```python
from build123d import *

# Parameters (mm, degrees)
SKETCH_1_R           = 2
EXTRUDE_1_DEPTH      = 6
CHAMFER_3_SIZE       = 2
SKETCH_4_R           = 4.2
EXTRUDE_2_DEPTH      = 6
SKETCH_7_R           = 8
EXTRUDE_3_DEPTH      = 7
FILLET_1_R           = 2
EXTRUDE_4_DEPTH      = 3
EXTRUDE_4_DEPTH_BACK = 3
SKETCH_9_R           = 4.2
CUT_EXTRUDE_1_DEPTH  = 10


with BuildPart() as part:
    # Эскиз1 → Бобышка-Вытянуть1 (new body)
    with BuildSketch(Plane(origin=(0, 0, 0), x_dir=(1, 0, 0), z_dir=(0, 1, 0))):
        with BuildLine():
            Line((0, -20), (0, 20))
            Line((0, 20), (-10.861288353, 20))
            ThreePointArc((-10.861288353, 20), (-12.418498887, 19.751325642), (-13.820814088, 19.030038141))
            Line((-13.820814088, 19.030038141), (-34.246577377, 4.030038141))
            ThreePointArc((-34.246577377, 4.030038141), (-36.287051642, 0), (-34.246577377, -4.030038141))
            Line((-34.246577377, -4.030038141), (-13.820814088, -19.030038141))
            ThreePointArc((-13.820814088, -19.030038141), (-12.418498887, -19.751325642), (-10.861288353, -20))
            Line((-10.861288353, -20), (0, -20))
        make_face()
        with Locations((-31.287051642, 0)):
            Circle(SKETCH_1_R, mode=Mode.SUBTRACT)
        with Locations((-10.861288353, -15)):
            Circle(SKETCH_1_R, mode=Mode.SUBTRACT)
        with Locations((-10.861288353, 15)):
            Circle(SKETCH_1_R, mode=Mode.SUBTRACT)
    extrude(amount=EXTRUDE_1_DEPTH)

    # Фаска3
    chamfer_3_edges = [part.edges().sort_by_distance(p)[0] for p in [
        (-12.861288353, 6, -15),
        (-33.287051642, 6, 0),
        (-12.861288353, 6, 15),
    ]]
    chamfer(chamfer_3_edges, length=CHAMFER_3_SIZE)

    # Эскиз4 → Бобышка-Вытянуть2 (add)
    with BuildSketch(Plane(origin=(0, 0, 0), x_dir=(0, 0, -1), z_dir=(1, 0, 0))):
        with BuildLine():
            Line((-7.252328736, 33.376940613), (-20, 6))
            Line((-20, 6), (20, 6))
            Line((20, 6), (7.252328736, 33.376940613))
            ThreePointArc((7.252328736, 33.376940613), (0, 38), (-7.252328736, 33.376940613))
        make_face()
        with Locations((0, 30)):
            Circle(SKETCH_4_R, mode=Mode.SUBTRACT)
    extrude(amount=-EXTRUDE_2_DEPTH)

    # Эскиз7 → Бобышка-Вытянуть3 (add)
    with BuildSketch(Plane.ZY.offset(6)):
        with Locations((0, 30)):
            Circle(SKETCH_7_R)
    extrude(amount=EXTRUDE_3_DEPTH)

    # Скругление1
    fillet_1_edges = [part.edges().sort_by_distance(p)[0] for p in [
        (-13, 30, -8),
    ]]
    fillet(fillet_1_edges, radius=FILLET_1_R)

    # Эскиз8 → Бобышка-Вытянуть4 (add, two sides)
    with BuildSketch(Plane.XY) as extrude_4_sk:
        Polygon((-26.427051642, 6), (-12.606919313, 30.486720465), (-11.530283794, 30.486720465), (-11.530283794, 17.734425211), (-4.808903741, 17.734425211), (-4.214748598, 6), align=None)
    extrude(amount=EXTRUDE_4_DEPTH)
    extrude(extrude_4_sk.sketch, amount=-EXTRUDE_4_DEPTH_BACK)

    # Эскиз9 → Вырез-Вытянуть1 (cut)
    with BuildSketch(Plane(origin=(0, 0, 0), x_dir=(0, 0, -1), z_dir=(1, 0, 0))):
        with Locations((0, 30)):
            Circle(SKETCH_9_R)
    extrude(amount=-CUT_EXTRUDE_1_DEPTH, mode=Mode.SUBTRACT)


solid = part.part
```
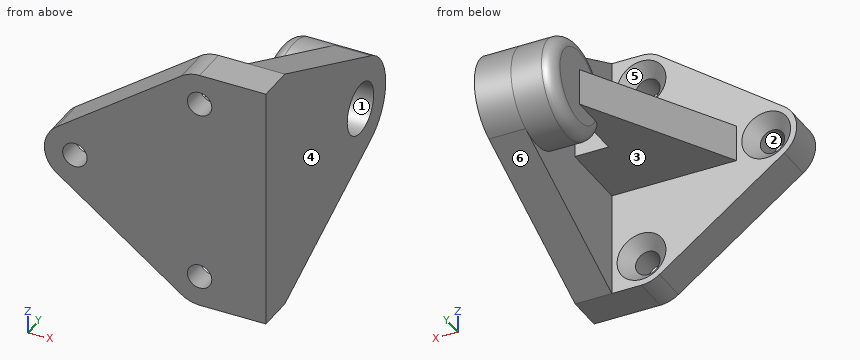
Here's how the part is built. I have some questions about the finished solid (model axes, mm). Face numbers are marked on the shaded views. A direction names the side the tool comes from. Coordinates: 2 decimals unless noted, no trailing zeros. Order: outer loops, then holes, each group sorted by start corner. A loop starts at its lowest first (then second) coordinate and runs counter-clockwise, first axis right, second up. Notation, with made-up numbers: (26, 55) - (69, 55) arc R15 ccw to (69, 59) - close; hole circle Ø11 at (71.5, -5.75). An arc over 180 degrees is marked (long way). One line per question, with ' | ' between items. Start each with the question number.
1. If we section it at D-D (y = 16.5): Write out the boundary of the cut face in (x, z).
2. If we section it at C-C (x = -8): Give the number of separate pieces and of enclosed holes in the cut face, and give its area (3 significant figures).
3. I'm going to push flat-ended pins straight in: pin 1 Ø1.5 at (y, z) = (15, -9) entering from +X; pin 2 Ø6.5 at (y, z) = (30, 0) entering from +X; pin 3 Ø3 at (y, z) = (21.5, 4) entering from -X; pin 4 Ø16.5 at (x, y) = (-17.5, 12) entering from -Z. Where does each tip first touch, or does it pass through?
4. Which directions (+Z, -Z, +X, -X, +Y, -Y) give clear straight access to the entire face, cutting with the end or side of a thin tool? Please do the marked faces 1, 2 and 3.
5. If we section it at A-A (z = 0): Write out the boundary of the cut face in (x, y), and give its area (3 significant figures).
6. Please list where these lines run through material, in increasing order: line 1 along Y through (x, z) = (-7.25, 0); line 2 along X through (y, z) = (1, 0); line 3 along X through (y, z) = (28, -9). Write a range as [from, to].
7. If we mould it in two halves opening along Z, with no side actions, what happens to the marked faces 4, 5 and 6? For each: released by +Z, released by -Z, zero draft, split by the parting line, or undercut.
8. If we section it at B-B (z = 15): Write out the boundary of the cut face in (x, y), and give its area (3 significant figures).
Model answer:
1) outline: (-20.5, -3) - (-6, -3) - (-6, -15.11) - (0, -15.11) - (0, 15.11) - (-6, 15.11) - (-6, 3) - (-20.5, 3) - close
2) separate pieces: 2 | enclosed holes: 1 | area: 448 mm²
3) pin 1: stops at x = 0 | pin 2: stops at x = -10 | pin 3: stops at x = -18.31 | pin 4: stops at z = -19.9
4) face 1: +X | face 2: +Y, -Y | face 3: -Z, -X
5) outline: (-36.29, 0) - (-33.29, 0) - (-33.29, 4) - (-35.29, 6) - (-36.29, 6) - close; (-29.29, 0) - (0, 0) - (0, 25.8) - (-10, 25.8) - (-10, 34.2) - (0, 34.2) - (0, 38) - (-11, 38) arc R2 ccw to (-13, 36) - (-13, 29.79) - (-26.43, 6) - (-27.29, 6) - (-29.29, 4) - close; hole (-11.53, 17.73) - (-6, 17.73) - (-6, 22) - (-11, 22) arc R2 cw to (-11.53, 22.07) - close | area: 657 mm²
6) line 1: y = [0, 17.73], [22, 25.8], [34.2, 38] | line 2: x = [-36.29, -33.29], [-29.29, 0] | line 3: x = [-6, 0]
7) face 4: zero draft | face 5: undercut | face 6: released by -Z
8) outline: (-19.31, 0) - (-12.86, 0) - (-12.86, 4) - (-14.86, 6) - (-19.31, 6) - close; (-8.86, 0) - (0, 0) - (0, 16.74) - (-6, 16.74) - (-6, 6) - (-6.86, 6) - (-8.86, 4) - close | area: 152 mm²
